Verification items for the finished model (mm, model axes). Face numbers are marked on the shaded views. A direction names the side the tool comes from. Give positions to 0.01 mm unless a question says otherwise; leave off trailing zeros. Order: outer loops, then holes, each group sorted by start corner. A loop starts at its lowest first (then second) coordinate and runs counter-clockwise, first axis right, second up.
(1) Access from +Z, -Z, +X, -X, +Y, -Y to the whole of each face (thin tool, end or side, straight path). Record for the marked faces 1, 2 and 3.
(2) Sectioned sample at C-C on z = -2.25. Record the cut outline in (x, y), plus the area to 3 significant figures.
(3) Mould release check, pull along Y, two halves, no side actions. Record for the marked faces 4, 5 and 6: pulls with the +Y half, pulls with the -Y half, needs draft (parallel to the pull), parting line crosses it, or undercut.
(4) Sectioned sample at B-B on y = -6. Record the cut outline in (x, z), plus the area to 3 significant figures.
(5) Gauge pin test, flat ends, axial feed: pin 1 (1.3 mm diameter, centred on y = 6, z = 1, fed in from -X); pin 2 (1.5 mm diameter, centred on y = 7, z = -3.5, fed in from -X); pin 3 (0.6 mm diameter, centred on x = 0.5, z = -4.5, fed in from +Y); pin 4 (0.6 mm diameter, centred on y = 12.5, z = -2.5, fed in from -X). Record the tip position at first contact, or that the pin passes through.
(6) Scan lines: L1, parallel to Y at x = 0, z = -2.15; L2, parallel to Y at x = -6.35, z = -1.75; L3, parallel to X at y = 0, z = 0.5. Record each from-to range of solid material in increasing order.
(7) Sectioned sample at D-D on y = -16. Record the cut outline in (x, z).
(8) Sectioned sample at A-A on x = 0. Count the separate pieces of the cut face and the enclosed holes in it, plus the area to 3 significant figures.
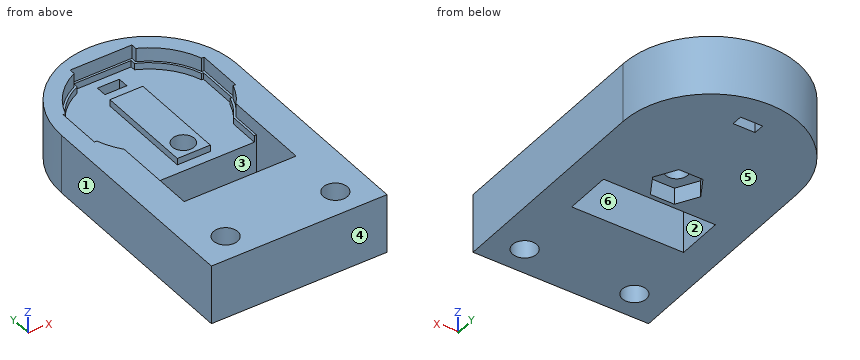
```python
from build123d import *

# Parameters (mm, degrees)
BOSS_EXTRUDE1_DEPTH     = 1.5875
SKETCH3_W               = 3.81
SKETCH3_H               = 11.43
BOSS_EXTRUDE2_DEPTH     = 0.762
SKETCH4_W               = 12.954
SKETCH4_H               = 1.3208
BOSS_EXTRUDE3_DEPTH     = 0.508
SKETCH5_W               = 12.954
SKETCH5_H               = 5.3848
BOSS_EXTRUDE4_DEPTH     = 4.5085
SKETCH2_R               = 1.27
CUT_EXTRUDE1_DEPTH      = 20.612110439
CUT_EXTRUDE1_DEPTH_BACK = 20.612110439
CUT_EXTRUDE2_DEPTH      = 1.905
SKETCH7_W               = 20.32
SKETCH7_H               = 6.9342
BOSS_EXTRUDE5_DEPTH     = 6.858
SKETCH8_R               = 1.397
CUT_EXTRUDE3_DEPTH      = 24.146480805
SKETCH9_W               = 2.54
SKETCH9_H               = 1.27
CUT_EXTRUDE4_DEPTH      = 24.146480805


with BuildPart() as part:
    # Sketch1 → Boss-Extrude1 (new body)
    with BuildSketch(Plane.XY):
        with BuildLine():
            Line((-10.16, 5.7658), (-10.16, -12.7))
            Line((-10.16, -12.7), (10.16, -12.7))
            Line((10.16, -12.7), (10.16, 5.7658))
            ThreePointArc((10.16, 5.7658), (0, 15.9258), (-10.16, 5.7658))
        make_face()
        with BuildLine():
            Line((-8.1661, 8.4328), (-8.1661, 3.0988))
            Line((-8.1661, 3.0988), (-7.88607878, 3.0988))
            ThreePointArc((-7.88607878, 3.0988), (-7.294970241, 1.754997498), (-6.477, 0.535924426))
            Line((-6.477, 0.535924426), (-6.477, -9.624254818))
            Line((-6.477, -9.624254818), (6.477, -9.624254818))
            Line((6.477, -9.624254818), (6.477, 0.535924426))
            ThreePointArc((6.477, 0.535924426), (7.294970241, 1.754997498), (7.88607878, 3.0988))
            Line((7.88607878, 3.0988), (8.1661, 3.0988))
            Line((8.1661, 3.0988), (8.1661, 8.4328))
            Line((8.1661, 8.4328), (7.88607878, 8.4328))
            ThreePointArc((7.88607878, 8.4328), (6.220422148, 11.298383105), (3.5687, 13.286937403))
            Line((3.5687, 13.286937403), (3.5687, 13.946945182))
            Line((3.5687, 13.946945182), (-3.5687, 13.946945182))
            Line((-3.5687, 13.946945182), (-3.5687, 13.286937403))
            ThreePointArc((-3.5687, 13.286937403), (-6.220422148, 11.298383105), (-7.88607878, 8.4328))
            Line((-7.88607878, 8.4328), (-8.1661, 8.4328))
        make_face(mode=Mode.SUBTRACT)
    extrude(amount=BOSS_EXTRUDE1_DEPTH)

    # Sketch3 → Boss-Extrude2 (add)
    with BuildSketch(Plane(origin=(0, 0, 0), x_dir=(-1, 0, 0), z_dir=(0, 0, -1))):
        with BuildLine():
            Line((-10.16, -12.7), (10.16, -12.7))
            Line((10.16, -12.7), (10.16, 5.7658))
            ThreePointArc((10.16, 5.7658), (0, 15.9258), (-10.16, 5.7658))
            Line((-10.16, 5.7658), (-10.16, -12.7))
        make_face()
        with BuildLine():
            Line((-6.477, -9.624254818), (-6.477, -2.918654818))
            Line((-6.477, -2.918654818), (-6.223, -2.918654818))
            Line((-6.223, -2.918654818), (-6.223, 0.535924426))
            Line((-6.223, 0.535924426), (-6.223, 0.626452695))
            ThreePointArc((-6.223, 0.626452695), (-7.094540168, 1.917927921), (-7.70169142, 3.3528))
            Line((-7.70169142, 3.3528), (-7.9121, 3.3528))
            Line((-7.9121, 3.3528), (-7.9121, 8.1788))
            Line((-7.9121, 8.1788), (-7.70169142, 8.1788))
            ThreePointArc((-7.70169142, 8.1788), (-6.037827534, 11.121475344), (-3.3147, 13.124562371))
            Line((-3.3147, 13.124562371), (-3.3147, 13.692945182))
            Line((-3.3147, 13.692945182), (3.3147, 13.692945182))
            Line((3.3147, 13.692945182), (3.3147, 13.124562371))
            ThreePointArc((3.3147, 13.124562371), (6.037827534, 11.121475344), (7.70169142, 8.1788))
            Line((7.70169142, 8.1788), (7.9121, 8.1788))
            Line((7.9121, 8.1788), (7.9121, 3.3528))
            Line((7.9121, 3.3528), (7.70169142, 3.3528))
            ThreePointArc((7.70169142, 3.3528), (7.094540168, 1.917927921), (6.223, 0.626452695))
            Line((6.223, 0.626452695), (6.223, -2.918654818))
            Line((6.223, -2.918654818), (6.477, -2.918654818))
            Line((6.477, -2.918654818), (6.477, -9.624254818))
            Line((6.477, -9.624254818), (-6.223, -9.624254818))
            Line((-6.223, -9.624254818), (-6.477, -9.624254818))
        make_face(mode=Mode.SUBTRACT)
        with Locations((0, 3.939345182)):
            Rectangle(SKETCH3_W, SKETCH3_H)
    extrude(amount=BOSS_EXTRUDE2_DEPTH)


with BuildPart() as boss_extrude2_piece_1:
    # of the separate pieces the step leaves, piece 1, a body of its own (boss_extrude2_pieces)
    add(part.part.solids().sort_by_distance((-10.16, 5.7658, 1.5875))[0])

    # Sketch4 → Boss-Extrude3 (add)
    with BuildSketch(Plane(origin=(0, 0, -0.762), x_dir=(-1, 0, 0), z_dir=(0, 0, -1))):
        with Locations((0, -8.963854818)):
            Rectangle(SKETCH4_W, SKETCH4_H)
    extrude(amount=-BOSS_EXTRUDE3_DEPTH)



with BuildPart() as boss_extrude2_piece_2:
    # of the separate pieces the step leaves, piece 2, a body of its own (boss_extrude2_pieces)
    add(part.part.solids().sort_by_distance((-1.905, -1.775654818, 0))[0])


with BuildPart() as boss_extrude2_piece_1_1:
    add(boss_extrude2_piece_1.part)

    add(boss_extrude2_piece_2.part)  # Boss-Extrude4 merges Boss-Extrude2 piece 2
    # Sketch5 → Boss-Extrude4 (add)
    with BuildSketch(Plane(origin=(0, 0, -0.762), x_dir=(-1, 0, 0), z_dir=(0, 0, -1))):
        with BuildLine():
            Line((10.16, -12.7), (10.16, 5.7658))
            ThreePointArc((10.16, 5.7658), (0, 15.9258), (-10.16, 5.7658))
            Line((-10.16, 5.7658), (-10.16, -12.7))
            Line((-10.16, -12.7), (10.16, -12.7))
        make_face()
        with Locations((0, -5.611054818)):
            Rectangle(SKETCH5_W, SKETCH5_H, mode=Mode.SUBTRACT)
    extrude(amount=BOSS_EXTRUDE4_DEPTH)

    # Sketch2 → Cut-Extrude1 (cut, two sides)
    with BuildSketch(Plane.XY) as cut_extrude1_sk:
        Circle(SKETCH2_R)
    extrude(amount=CUT_EXTRUDE1_DEPTH, mode=Mode.SUBTRACT)
    extrude(cut_extrude1_sk.sketch, amount=-CUT_EXTRUDE1_DEPTH_BACK, mode=Mode.SUBTRACT)

    # Sketch6 → Cut-Extrude2 (cut)
    with BuildSketch(Plane(origin=(0, 0, -5.2705), x_dir=(-1, 0, 0), z_dir=(0, 0, -1))):
        Polygon((1.3931462, 2.413), (-1.3931462, 2.413), (-2.786292399, 0), (-1.3931462, -2.413), (1.3931462, -2.413), (2.786292399, 0), align=None)
    extrude(amount=-CUT_EXTRUDE2_DEPTH, mode=Mode.SUBTRACT)

    # Sketch7 → Boss-Extrude5 (add)
    with BuildSketch(Plane(origin=(0, 0, -5.2705), x_dir=(-1, 0, 0), z_dir=(0, 0, -1))):
        with Locations((0, -16.1671)):
            Rectangle(SKETCH7_W, SKETCH7_H)
    extrude(amount=-BOSS_EXTRUDE5_DEPTH)

    # Sketch8 → Cut-Extrude3 (cut, through all)
    with BuildSketch(Plane(origin=(0, 0, -5.2705), x_dir=(-1, 0, 0), z_dir=(0, 0, -1))):
        with Locations((-6.35, -16.4592)):
            Circle(SKETCH8_R)
        with Locations((6.35, -16.4592)):
            Circle(SKETCH8_R)
    extrude(amount=-CUT_EXTRUDE3_DEPTH, mode=Mode.SUBTRACT)

    # Sketch9 → Cut-Extrude4 (cut, through all)
    with BuildSketch(Plane(origin=(0, 0, -5.2705), x_dir=(-1, 0, 0), z_dir=(0, 0, -1))):
        with Locations((0, 12.065)):
            Rectangle(SKETCH9_W, SKETCH9_H)
    extrude(amount=-CUT_EXTRUDE4_DEPTH, mode=Mode.SUBTRACT)


solid = boss_extrude2_piece_1_1.part
```
Ans:
1. face 1: +Z, -Z, -X, +Y, -Y
1. face 2: +Z
1. face 3: +Z, -Z
2. outline: (-10.16, -19.63) - (10.16, -19.63) - (10.16, 5.77) arc R10.16 ccw to (-10.16, 5.77) - close; hole circle Ø2.79 at (-6.35, -16.46); hole (-6.48, -8.3) - (6.48, -8.3) - (6.48, -2.92) - (-6.48, -2.92) - close; hole circle Ø2.54 at (0, 0); hole (-1.27, 11.43) - (1.27, 11.43) - (1.27, 12.7) - (-1.27, 12.7) - close; hole circle Ø2.79 at (6.35, -16.46)
2. area: 588 mm2
3. face 4: pulls with the -Y half
3. face 5: needs draft
3. face 6: undercut
4. outline: (-10.16, -5.27) - (-6.48, -5.27) - (-6.48, 1.59) - (-10.16, 1.59) - close; (6.48, -5.27) - (10.16, -5.27) - (10.16, 1.59) - (6.48, 1.59) - close
4. area: 50.5 mm2
5. pin 1: stops at x = -10.16
5. pin 2: stops at x = -10.15
5. pin 3: stops at y = 15.92
5. pin 4: stops at x = -7.86
6. L1: y = -19.63 to -8.3, -2.92 to -1.27, 1.27 to 11.43, 12.7 to 15.93
6. L2: y = -19.63 to -17.86, -15.06 to -8.3, -2.92 to 13.7
6. L3: x = -10.16 to -6.48, 6.48 to 10.16
7. outline: (-10.16, -5.27) - (-7.67, -5.27) - (-7.67, 1.59) - (-10.16, 1.59) - close; (-5.03, -5.27) - (5.03, -5.27) - (5.03, 1.59) - (-5.03, 1.59) - close; (7.67, -5.27) - (10.16, -5.27) - (10.16, 1.59) - (7.67, 1.59) - close
8. separate pieces: 4
8. enclosed holes: 0
8. area: 150 mm2
